Build history of the part. All positions in model axes, mm. Face numbers are marked on the shaded views. Round coordinates to 2 decimals unless told otherwise and drop trailing zeros. Write each loop counter-clockwise with the first axis right and the second up, starting at its lowest first coordinate (ties: lowest second). Pieces come first, ordered by that corner, then holes. Notation, with made-up numbers: (0, 62.5) -> (58, 62.5) arc R21 ccw to (58, 88.5) -> close; hole circle Ø1 at (-24, -4). An arc over 180 degrees is marked (long way). Return JSON: item names as keys, results as strings.
from build123d import *

# Parameters (mm, degrees)
SKETCH1_R           = 2.5
BOSS_EXTRUDE1_DEPTH = 5
FILLET1_R           = 10
FILLET2_R           = 5


with BuildPart() as part:
    # Sketch1 → Boss-Extrude1 (new body)
    with BuildSketch(Plane.XY):
        Polygon((0, 0), (0, 40), (-20.152940401, 60.152940401), (-6.010804777, 74.295076025), (20, 48.284271247), (20, 0), align=None)
        with Locations((10, 10)):
            Circle(SKETCH1_R, mode=Mode.SUBTRACT)
        with Locations((10, 35)):
            Circle(SKETCH1_R, mode=Mode.SUBTRACT)
        with Locations((-4.419570665, 58.561706289)):
            Circle(SKETCH1_R, mode=Mode.SUBTRACT)
    extrude(amount=BOSS_EXTRUDE1_DEPTH)

    # Fillet1
    fillet1_edges = [part.edges().sort_by_distance(p)[0] for p in [
        (20, 48.284271247, 2.5),
        (0, 40, 2.5),
        (-20.152940401, 60.152940401, 2.5),
        (-6.010804777, 74.295076025, 2.5),
    ]]
    fillet(fillet1_edges, radius=FILLET1_R - 0.0001)  # a hair under: the kernel refuses the full size

    # Fillet2
    fillet2_edges = [part.edges().sort_by_distance(p)[0] for p in [
        (0, 0, 2.5),
        (20, 0, 2.5),
    ]]
    fillet(fillet2_edges, radius=FILLET2_R)


solid = part.part
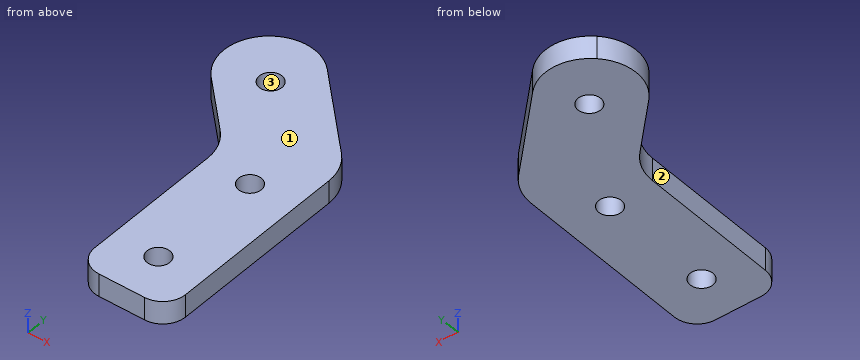
Q1. Saw through at D-D on x = -12. List the corners of the cut face in (y, z).
Verdict:
{"outline": "(52, 0) -> (68.16, 0) -> (68.16, 5) -> (52, 5) -> close"}
Q2. Pin check, flat tips, straight feed: pin 1 Ø2.5 at (y, z) = (26.5, 3.5) entering from -X; pin 2 Ø8 at (x, y) = (-4.42, 58.56) entering from +Z; pin 3 Ø1.5 at (y, z) = (38.5, 3) entering from -X; pin 4 Ø1 at (x, z) = (11, 1) entering from +Y. Stop position of each tip, or through.
Verdict:
{"pin 1": "stops at x = 0", "pin 2": "stops at z = 5", "pin 3": "stops at x = -0.59", "pin 4": "stops at y = 57.78"}
Q3. Wall check: L1, parallel to Y at x = 10, z = 2.1; L2, parallel to X at y = 27.5, z = 0.6; L3, parallel to Y at x = -3, z = 4.85. Give the ranges that are in metal, low to high.
Verdict:
{"L1": "y = 0 to 7.5, 12.5 to 32.5, 37.5 to 58.28", "L2": "x = 0 to 20", "L3": "y = 43 to 56.5, 60.62 to 69.69"}
Q4. Saw through at A-A on y = 35. List the corners of the cut face in (x, z).
Verdict:
{"outline": "(0, 0) -> (7.5, 0) -> (7.5, 5) -> (0, 5) -> close; (12.5, 0) -> (20, 0) -> (20, 5) -> (12.5, 5) -> close"}
Q5. Saw through at B-B on z = 2.85. Count the separate pieces of the cut face and the enclosed holes in it, then the cut area to 3 significant figures.
Verdict:
{"separate pieces": "1", "enclosed holes": "3", "area": "1,420 mm²"}
Q6. Two-plate mould, pull along X, no slides. Class the marked faces 1, 2 and 3: +X half, -X half, draft (parallel to the pull), parting line (faces both ways), or undercut.
Verdict:
{"face 1": "draft", "face 2": "-X half", "face 3": "undercut"}
Q7. Saw through at C-C on x = 10. List the corners of the cut face in (y, z), then the cut area to 3 significant figures.
Verdict:
{"outline": "(0, 0) -> (7.5, 0) -> (7.5, 5) -> (0, 5) -> close; (12.5, 0) -> (32.5, 0) -> (32.5, 5) -> (12.5, 5) -> close; (37.5, 0) -> (58.28, 0) -> (58.28, 5) -> (37.5, 5) -> close", "area": "241 mm²"}
